Geometry check sheet. Reference: the model listing, model coordinates, mm. Face numbers are marked on the shaded views. A direction names the side the tool comes from. Coordinates: 2 decimals unless noted, no trailing zeros. Order: outer loops, then holes, each group sorted by start corner. A loop starts at its lowest first (then second) coordinate and runs counter-clockwise, first axis right, second up. Notation, with made-up numbers: (32.5, -38.75) - (66.5, -38.75) arc R21 cw to (66.5, -16.75) - close; hole circle Ø7 at (-38.75, 86). An arc over 180 degrees is marked (long way). Put each result on its own line as item: value.
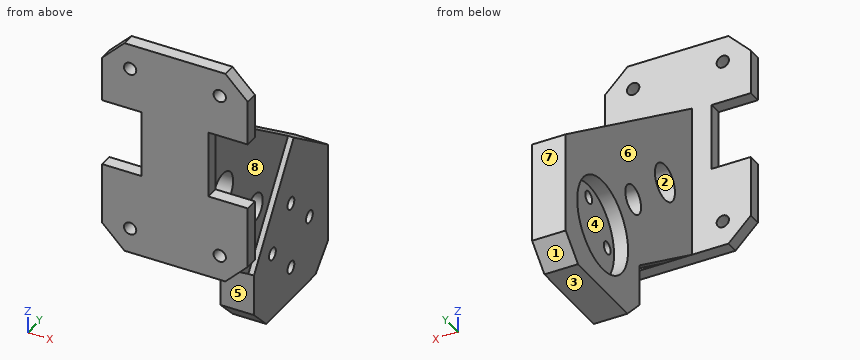
from build123d import *

# Parameters (mm, degrees)
EXTRUDE_1_DEPTH      = 30
SKETCH_2_R           = 8.25
CUT_EXTRUDE_1_DEPTH  = 2.5
EXTRUDE_2_DEPTH      = 41
SKETCH_6_R           = 8
CUT_EXTRUDE_3_DEPTH  = 4
CUT_EXTRUDE_4_DEPTH  = 83.710337927
CUT_EXTRUDE_6_DEPTH  = 23
EXTRUDE_3_DEPTH      = 23
CUT_EXTRUDE_7_DEPTH  = 46.5
EXTRUDE_4_DEPTH      = 4
CUT_EXTRUDE_8_DEPTH  = 23
CUT_EXTRUDE_9_DEPTH  = 65.964988157
SKETCH_16_R          = 1.25
CUT_EXTRUDE_10_DEPTH = 65.964988157
CUT_EXTRUDE_11_DEPTH = 44
EXTRUDE_5_DEPTH      = 2.5
CUT_EXTRUDE_12_DEPTH = 3
EXTRUDE_6_DEPTH      = 41
CUT_EXTRUDE_13_DEPTH = 41
CUT_EXTRUDE_14_DEPTH = 17
CHAMFER_1_SIZE       = 4
CUT_EXTRUDE_16_DEPTH = 53.085522264
EXTRUDE_8_DEPTH      = 5
CUT_EXTRUDE_17_DEPTH = 4
SKETCH_30_W          = 26
SKETCH_30_H          = 39
SKETCH_30_R          = 1.1
EXTRUDE_10_DEPTH     = 2.3
CHAMFER_4_SIZE       = 4
SKETCH_32_R          = 2.551786445
SKETCH_32_R_2        = 3.249198584
CUT_EXTRUDE_18_DEPTH = 48.085687781
SKETCH_33_W          = 7
SKETCH_33_H          = 12
CUT_EXTRUDE_19_DEPTH = 10
EXTRUDE_11_DEPTH     = 1
SKETCH_8_R           = 1.1
CUT_EXTRUDE_5_DEPTH  = 47.322910032


with BuildPart() as part:
    # 草图1 → 凸台-拉伸1 (new body)
    with BuildSketch(Plane(origin=(0, 0, 0), x_dir=(1, 0, 0), z_dir=(0, 1, 0))):
        Polygon((0, 0), (-15.325055808, 0), (-21.84047557, -15.349367059), (5.774670034, -27.071300914), (30, 30), (0, 30), align=None)
    extrude(amount=EXTRUDE_1_DEPTH)

    # 草图2 → 切除-拉伸1 (cut)
    with BuildSketch(Plane.ZY):
        with Locations((-15, 15)):
            Circle(SKETCH_2_R)
    extrude(amount=-CUT_EXTRUDE_1_DEPTH, mode=Mode.SUBTRACT)

    # 草图5 → 凸台-拉伸2 (add)
    with BuildSketch(Plane.XZ):
        Polygon((-21.84047557, 15.349367059), (-9.337079458, -14.106788251), (18.278066145, -2.384854396), (5.774670034, 27.071300914), align=None)
    extrude(amount=EXTRUDE_2_DEPTH)

    # 草图6 → 切除-拉伸3 (cut)
    with BuildSketch(Plane.XZ.offset(41)):
        with Locations(Location((-1.781204712, 6.482256331, 0), (0, 0, 270))):
            Circle(SKETCH_6_R)
    extrude(amount=-CUT_EXTRUDE_3_DEPTH, mode=Mode.SUBTRACT)

    # 草图7 → 切除-拉伸4 (cut, through all)
    with BuildSketch(Plane(origin=(0, 30, 0), x_dir=(1, 0, 0), z_dir=(0, 1, 0))):
        Polygon((0, 27), (5, 27), (5, -28.896309146), (30, 30), (0, 30), align=None)
    extrude(amount=-CUT_EXTRUDE_4_DEPTH, mode=Mode.SUBTRACT)

    # 草图10 → 切除-拉伸6 (cut)
    with BuildSketch(Plane.XZ.offset(41)):
        Polygon((-19.999465863, 16.130829316), (-7.496069751, -13.325325994), (-9.337079458, -14.106788251), (-21.84047557, 15.349367059), align=None)
        Polygon((5.774670034, 27.071300914), (3.933660327, 26.289838657), (16.437056438, -3.166316653), (18.278066145, -2.384854396), align=None)
    extrude(amount=-CUT_EXTRUDE_6_DEPTH, mode=Mode.SUBTRACT)

    # 草图11 → 凸台-拉伸3 (add)
    with BuildSketch(Plane.XZ.offset(41)):
        Polygon((-19.999465863, 16.130829316), (-24.297508276, 26.256382704), (-0.364382087, 36.415392045), (3.933660327, 26.289838657), align=None)
        Polygon((5, 23.777699815), (16.437056438, -3.166316653), (5, -8.021059083), align=None)
    extrude(amount=-EXTRUDE_3_DEPTH)

    # 草图12 → 切除-拉伸7 (cut)
    with BuildSketch(Plane.XZ.offset(41)):
        Polygon((0.345866355, -31.799769722), (-9.058994265, -9.64330658), (14.874131924, 0.51570276), (24.278992544, -21.640760381), align=None)
    extrude(amount=-CUT_EXTRUDE_7_DEPTH, mode=Mode.SUBTRACT)

    # 草图13 → 凸台-拉伸4 (add)
    with BuildSketch(Plane(origin=(0, -18, 0), x_dir=(1, 0, 0), z_dir=(0, 1, 0))):
        Polygon((14.874131924, -0.51570276), (-9.058994265, 9.64330658), (-24.297508276, -26.256382704), (-0.364382087, -36.415392045), align=None)
    extrude(amount=EXTRUDE_4_DEPTH)

    # 草图14 → 切除-拉伸8 (cut)
    with BuildSketch(Plane.XZ.offset(41)):
        Polygon((-9.058994265, -9.64330658), (14.874131924, 0.51570276), (-0.364382087, 36.415392045), (-24.297508276, 26.256382704), align=None)
    extrude(amount=-CUT_EXTRUDE_8_DEPTH, mode=Mode.SUBTRACT)

    # 草图15 → 切除-拉伸9 (cut, through all)
    with BuildSketch(Plane.XZ.offset(18)):
        Polygon((5, 23.777699815), (5, 26.742472994), (3.933660327, 26.289838657), align=None)
        Polygon((-19.999465863, 16.130829316), (-7.496069751, -13.325325994), (-9.337079458, -14.106788251), (-21.84047557, 15.349367059), align=None)
    extrude(amount=-CUT_EXTRUDE_9_DEPTH, mode=Mode.SUBTRACT)

    # 草图16 → 切除-拉伸10 (cut, through all)
    with BuildSketch(Plane.XZ.offset(18)):
        with Locations(Location((-17.936693931, 24.067766506, 0), (0, 0, 270))):
            Circle(SKETCH_16_R)
        with Locations(Location((-3.208616276, 30.319464562, 0), (0, 0, 90))):
            Circle(SKETCH_16_R)
        with Locations(Location((8.513317579, 2.704318958, 0), (0, 0, 270))):
            Circle(SKETCH_16_R)
        with Locations(Location((-6.214760076, -3.547379097, 0), (0, 0, 270))):
            Circle(SKETCH_16_R)
    extrude(amount=-CUT_EXTRUDE_10_DEPTH, mode=Mode.SUBTRACT)

    # 草图17 → 切除-拉伸11 (cut)
    with BuildSketch(Plane(origin=(0, 30, 0), x_dir=(1, 0, 0), z_dir=(0, 1, 0))):
        Polygon((-9.058994265, 9.64330658), (-19.999465863, -16.130829316), (0, -24.620098913), (0, 5.797991655), align=None)
    extrude(amount=-CUT_EXTRUDE_11_DEPTH, mode=Mode.SUBTRACT)

    # 草图18 → 凸台-拉伸5 (add)
    with BuildSketch(Plane.XZ.offset(-5.5)):
        Polygon((5, -3.675617573), (0, -5.797991655), (0, -27), (5, -27), align=None)
    extrude(amount=EXTRUDE_5_DEPTH)

    # 草图20 → 切除-拉伸12 (cut)
    with BuildSketch(Plane(origin=(0, 30, 0), x_dir=(1, 0, 0), z_dir=(0, 1, 0))):
        Polygon((0, 27), (0, -24.620098913), (3.933660327, -26.289838657), (5, -23.777699815), (5, 27), align=None)
    extrude(amount=-CUT_EXTRUDE_12_DEPTH, mode=Mode.SUBTRACT)

    # 草图21 → 凸台-拉伸6 (add)
    with BuildSketch(Plane(origin=(0, 27, 0), x_dir=(1, 0, 0), z_dir=(0, 1, 0))):
        Polygon((0, -24.620098913), (0, -35.556961644), (3.933660327, -26.289838657), align=None)
    extrude(amount=-EXTRUDE_6_DEPTH)

    # 草图22 → 切除-拉伸13 (cut)
    with BuildSketch(Plane(origin=(0, 27, 0), x_dir=(1, 0, 0), z_dir=(0, 1, 0))):
        Polygon((5, -23.777699815), (0, -23.777699815), (0, -35.556961644), align=None)
    extrude(amount=-CUT_EXTRUDE_13_DEPTH, mode=Mode.SUBTRACT)

    # 草图23 → 切除-拉伸14 (cut)
    with BuildSketch(Plane.XZ.offset(-3)):
        Polygon((5, -3.675617573), (0, -3.675617573), (0, -5.797991655), align=None)
    extrude(amount=CUT_EXTRUDE_14_DEPTH, mode=Mode.SUBTRACT)

    # 倒角1
    chamfer_1_edges = [part.edges().sort_by_distance(p)[0] for p in [
        (-24.297508276, -16, 26.256382704),
        (-0.364382087, -16, 36.415392045),
        (14.874131924, -16, 0.51570276),
        (-9.058994265, -16, -9.64330658),
        (2.5, 3, -27),
        (2.5, 27, -27),
    ]]
    chamfer(chamfer_1_edges, length=CHAMFER_1_SIZE)

    # 草图26 → 切除-拉伸16 (cut, through all)
    with BuildSketch(Plane(origin=(5, 0, 0), x_dir=(0, 0, -1), z_dir=(1, 0, 0))):
        Polygon((-23.777699815, -14), (4.930809251, 27), (-23.777699815, 27), align=None)
    extrude(amount=-CUT_EXTRUDE_16_DEPTH, mode=Mode.SUBTRACT)

    # 草图27 → 凸台-拉伸8 (add)
    with BuildSketch(Plane(origin=(5, 0, 0), x_dir=(0, 0, -1), z_dir=(1, 0, 0))):
        Polygon((3.675617573, -14), (15.579145723, 3), (3.675617573, 3), align=None)
    extrude(amount=-EXTRUDE_8_DEPTH)

    # 草图31 → 切除-拉伸17 (cut)
    with BuildSketch(Plane.XZ.offset(18)):
        Polygon((-5.376974851, -8.080382066), (11.192112511, -1.047221754), (13.311207411, 4.197722174), (1.198542427, 32.733372631), (-4.0464015, 34.852467531), (-20.615488863, 27.819307218), (-22.734583762, 22.574363291), (-10.621918779, -5.961287167), align=None)
    extrude(amount=-CUT_EXTRUDE_17_DEPTH, mode=Mode.SUBTRACT)

    # 草图30 → 凸台-拉伸10 (add)
    with BuildSketch(Plane(origin=(0, -14, 0), x_dir=(1, 0, 0), z_dir=(0, 1, 0))):
        with Locations((2.5, -15.824382427)):
            Rectangle(SKETCH_30_W, SKETCH_30_H)
        with Locations(Location((-5.5, -0.824382427, 0), (0, 0, 270))):
            Circle(SKETCH_30_R, mode=Mode.SUBTRACT)
        with Locations(Location((10.5, -0.824382427, 0), (0, 0, 90))):
            Circle(SKETCH_30_R, mode=Mode.SUBTRACT)
        with Locations(Location((10.5, -30.824382427, 0), (0, 0, 270))):
            Circle(SKETCH_30_R, mode=Mode.SUBTRACT)
        with Locations(Location((-5.5, -30.824382427, 0), (0, 0, 90))):
            Circle(SKETCH_30_R, mode=Mode.SUBTRACT)
    extrude(amount=-EXTRUDE_10_DEPTH)

    # 倒角4
    chamfer_4_edges = [part.edges().sort_by_distance(p)[0] for p in [
        (-10.5, -15.15, 35.324382427),
        (-10.5, -15.15, -3.675617573),
        (15.5, -15.15, -3.675617573),
        (15.5, -15.15, 35.324382427),
    ]]
    chamfer(chamfer_4_edges, length=CHAMFER_4_SIZE)

    # 草图32 → 切除-拉伸18 (cut, through all)
    with BuildSketch(Plane.ZY):
        with Locations((-4.425551632, 5.088873795)):
            Circle(SKETCH_32_R)
        with Locations((4.800137825, -5.216417619)):
            Circle(SKETCH_32_R_2)
    extrude(amount=-CUT_EXTRUDE_18_DEPTH, mode=Mode.SUBTRACT)

    # 草图33 → 切除-拉伸19 (cut)
    with BuildSketch(Plane.XZ.offset(16.3)):
        with Locations((-7, 17.324382427)):
            Rectangle(SKETCH_33_W, SKETCH_33_H)
        with Locations((12, 17.324382427)):
            Rectangle(SKETCH_33_W, SKETCH_33_H)
    extrude(amount=-CUT_EXTRUDE_19_DEPTH, mode=Mode.SUBTRACT)

    # 草图34 → 凸台-拉伸11 (add)
    with BuildSketch(Plane(origin=(5, 0, 0), x_dir=(0, 0, -1), z_dir=(1, 0, 0))):
        Polygon((15.579145723, 3), (-2.842306745, 15.898839883), (4.930809251, 27), (23, 27), (27, 23), (27, 7), (23, 3), align=None)
    extrude(amount=EXTRUDE_11_DEPTH)

    # 草图8 → 切除-拉伸5 (cut, through all)
    with BuildSketch(Plane.ZY.offset(-2.5)):
        with Locations((-15, 21)):
            Circle(SKETCH_8_R)
        with Locations((-9, 15)):
            Circle(SKETCH_8_R)
        with Locations(Location((-15, 9, 0), (0, 0, 180))):
            Circle(SKETCH_8_R)
        with Locations(Location((-21, 15, 0), (0, 0, 180))):
            Circle(SKETCH_8_R)
    extrude(amount=-CUT_EXTRUDE_5_DEPTH, mode=Mode.SUBTRACT)


solid = part.part
Q1. Access from +Z, -Z, +X, -X, +Y, -Y to the whole of each face (thin tool, end or side, straight path). Record for the marked faces 4, 5, 6, 7 and 8.
Answer block:
face 4: -X
face 5: -Z, +X, -X, -Y
face 6: +Z, -Z, -X, +Y
face 7: +Z, -Z, +X, -X, +Y
face 8: +Z, +X
Q2. Section check B-B on x = -5.5. Record the boundary of the cut face in (y, z), then the cut area to 3 significant figures.
Answer block:
outline: (-16.3, -3.68) - (-14, -3.68) - (-14, -0.28) - (-16.3, -0.28) - close; (-16.3, 1.92) - (-14, 1.92) - (-14, 11.32) - (-16.3, 11.32) - close; (-16.3, 23.32) - (-14, 23.32) - (-14, 29.72) - (-16.3, 29.72) - close; (-16.3, 31.92) - (-14, 31.92) - (-14, 35.32) - (-16.3, 35.32) - close
area: 52.0 mm^2
Q3. Depth check by flat-ended pin: pin 1 Ø2.5 at (x, z) = (-5.5, 0.82) entering from +Y; pin 2 Ø1.2 at (x, y) = (7, -15) entering from -Z; pin 3 Ø2 at (x, y) = (3.5, 3.5) entering from +Z. Enter the tip coordinate at first touch or a pass-through.
Answer block:
pin 1: stops at y = -14
pin 2: stops at z = -3.68
pin 3: stops at z = 12.22
Q4. Section check D-D on z = 15.5. Record the boundary of the cut face in (x, y).
Answer block:
outline: (-3.5, -16.3) - (8.5, -16.3) - (8.5, -14) - (5, -14) - (5, -2.18) - (0, -2.18) - (0, -14) - (-3.5, -14) - close
Q5. Draft check along Y on the marked faces 1, 2 and 3. Enter one of: pulls with the +Y half, pulls with the -Y half, needs draft (parallel to the pull), parting line crosses it, or undercut.
Answer block:
face 1: pulls with the +Y half
face 2: undercut
face 3: needs draft
Q6. Section check A-A on y = 9. Record the boundary of the cut face in (x, z).
Answer block:
outline: (0, -27) - (6, -27) - (6, -16.1) - (2.5, -16.1) - (2.5, -20.66) - (0, -20.66) - close; (0, -9.34) - (2.5, -9.34) - (2.5, -13.9) - (6, -13.9) - (6, -7.01) - (5, -7.01) - (5, 7.67) - (0, 7.67) - close
Q7. Thickness scan on L1, parallel to Y at x = 4, z = -15; L2, parallel to X at y = 14.5, z = -1; L3, parallel to X at y = 3, z = 5.5. Record the ranges inside material, lowest first. Write a range as [from, to].
Answer block:
L1: y = [2.17, 7.9], [10.1, 19.9], [22.1, 27]
L2: x = [0, 6]
L3: x = [0, 5]
Q8. Section check C-C on z = -9. Record the boundary of the cut face in (x, y), then the cut area to 3 significant figures.
Answer block:
outline: (0, -6.4) - (5, -6.4) - (5, 7.61) - (6, 7.61) - (6, 13.9) - (2.5, 13.9) - (2.5, 9.34) - (0, 9.34) - close; (0, 20.66) - (2.5, 20.66) - (2.5, 16.1) - (6, 16.1) - (6, 27) - (0, 27) - close
area: 150 mm^2
